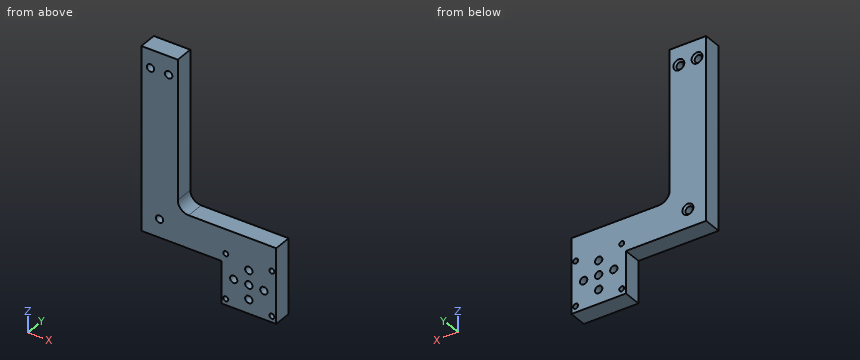
from build123d import *

# Parameters (mm, degrees)
BOSS_EXTRUDE1_DEPTH               = 12.7
F_1_4_20_TAPPED_HOLE1_D           = 5.1054
F_1_4_20_TAPPED_HOLE1_DEPTH       = 12.7
F_1_4_20_TAPPED_HOLE1_CSINK_D     = 7.62
F_1_4_20_TAPPED_HOLE1_CSINK_ANGLE = 90
F_1_4_20_TAPPED_HOLE2_D           = 5.1054
F_1_4_20_TAPPED_HOLE2_DEPTH       = 12.7
F_1_4_20_TAPPED_HOLE2_CSINK_D     = 7.62
F_1_4_20_TAPPED_HOLE2_CSINK_ANGLE = 90
F_29_0_136_DIAMETER_HOLE1_D       = 3.4544
F_29_0_136_DIAMETER_HOLE1_DEPTH   = 12.7
F_1_4_20_TAPPED_HOLE4_D           = 5.1054
F_1_4_20_TAPPED_HOLE4_DEPTH       = 12.7
LPATTERN1_COUNT                   = 3
LPATTERN1_PITCH                   = 10
F_1_4_20_TAPPED_HOLE6_D           = 5.1054
F_1_4_20_TAPPED_HOLE6_DEPTH       = 12.7
FILLET1_R                         = 7.62


with BuildPart() as part:
    # Sketch1 → Boss-Extrude1 (new body)
    with BuildSketch(Plane(origin=(0, 0, 0), x_dir=(1, 0, 0), z_dir=(0, 1, 0))):
        Polygon((81.28, 40.64), (81.28, 92.71), (43.18, 92.71), (43.18, 63.5), (12.7, 63.5), (-12.7, 63.5), (-12.7, -63.5), (12.7, -63.5), (12.7, 40.64), align=None)
    extrude(amount=BOSS_EXTRUDE1_DEPTH)

    # 1/4-20 Tapped Hole1
    with Locations(Plane(origin=(0, 12.7, 0), x_dir=(1, 0, 0), z_dir=(0, 1, 0))):
        with Locations((-6.35, -50.8), (6.35, -50.8)):
            CounterSinkHole(F_1_4_20_TAPPED_HOLE1_D / 2, F_1_4_20_TAPPED_HOLE1_CSINK_D / 2, depth=F_1_4_20_TAPPED_HOLE1_DEPTH, counter_sink_angle=F_1_4_20_TAPPED_HOLE1_CSINK_ANGLE)

    # 1/4-20 Tapped Hole2
    with Locations(Plane(origin=(0, 12.7, 0), x_dir=(1, 0, 0), z_dir=(0, 1, 0))):
        with Locations((0, 50.8)):
            CounterSinkHole(F_1_4_20_TAPPED_HOLE2_D / 2, F_1_4_20_TAPPED_HOLE2_CSINK_D / 2, depth=F_1_4_20_TAPPED_HOLE2_DEPTH, counter_sink_angle=F_1_4_20_TAPPED_HOLE2_CSINK_ANGLE)

    # #29 (0.136) Diameter Hole1
    with Locations(Plane(origin=(0, 12.7, 0), x_dir=(1, 0, 0), z_dir=(0, 1, 0))):
        with Locations((46.18, 88.44), (78.28, 88.44), (46.18, 57.44), (78.28, 57.44)):
            Hole(F_29_0_136_DIAMETER_HOLE1_D / 2, depth=F_29_0_136_DIAMETER_HOLE1_DEPTH)

    # 1/4-20 Tapped Hole4
    with Locations(Plane(origin=(0, 12.7, 0), x_dir=(1, 0, 0), z_dir=(0, 1, 0))):
        with Locations((62.23, 82.94)):
            f_1_4_20_tapped_hole4 = Hole(F_1_4_20_TAPPED_HOLE4_D / 2, depth=F_1_4_20_TAPPED_HOLE4_DEPTH)

    # LPattern1: 1/4-20 Tapped Hole4 ×3
    with Locations(*[(0, 0, i * LPATTERN1_PITCH) for i in range(1, LPATTERN1_COUNT)]):
        add(f_1_4_20_tapped_hole4, mode=Mode.SUBTRACT)

    # 1/4-20 Tapped Hole6
    with Locations(Plane(origin=(0, 12.7, 0), x_dir=(1, 0, 0), z_dir=(0, 1, 0))):
        with Locations((51.68, 72.972413119), (72.71230772, 72.972413119)):
            Hole(F_1_4_20_TAPPED_HOLE6_D / 2, depth=F_1_4_20_TAPPED_HOLE6_DEPTH)

    # Fillet1
    fillet1_edges = [part.edges().sort_by_distance(p)[0] for p in [
        (12.7, 6.35, -40.64),
    ]]
    fillet(fillet1_edges, radius=FILLET1_R)


solid = part.part
Geometry: final body of the model. Coordinates: model frame, mm. Coordinates: 2 decimals unless noted, no trailing zeros. Order: outer loops, then holes, each group sorted by start corner. A loop starts at its lowest first (then second) coordinate and runs counter-clockwise, first axis right, second up.
(1) Material intervals for probe 1 along X at (y, z) = (5, -57.44); probe 2 along Z at (x, y) = (62.5, 8.25); probe 3 along Z at (x, y) = (78.28, 7), sorted ascending.
(2) First-contact query: pin 1 (4.5 mm diameter, centred on x = 72.71, z = -72.97, fed in from -Y); pin 2 (6.5 mm diameter, centred on x = 25, y = 4.5, fed in from -Z); pin 3 (4 mm diameter, centred on x = 53, y = 7.5, fed in from +Z); pin 4 (6.5 mm diameter, centred on x = 6.35, z = 50.8, fed in from +Y). Flat tips, straight axial feed; report the tip coordinate or a pass-through.
(3) Section query C-C (x = -6.35). Return the cut outline in (y, z), plus the area to 3 significant figures.
(4) Section query B-B (x = 62.23). Return the cut outline in (y, z).
(5) Section query A-A (z = -88.44). Return the cut outline in (x, y), plus the area to 3 significant figures.
(6) Section query D-D (z = -57.44). Return the cut outline in (x, y).
Solution:
1. probe 1: x = -12.7 to 44.45, 47.91 to 76.55, 80.01 to 81.28
1. probe 2: z = -92.71 to -85.48, -80.4 to -75.48, -70.4 to -65.48, -60.4 to -40.64
1. probe 3: z = -92.71 to -90.17, -86.71 to -59.17, -55.71 to -40.64
2. pin 1: passes through
2. pin 2: stops at z = -63.5
2. pin 3: stops at z = -40.64
2. pin 4: stops at y = 12.14
3. outline: (0, -63.5) - (12.7, -63.5) - (12.7, 46.99) - (11.44, 48.25) - (0, 48.25) - close; (0, 53.35) - (11.44, 53.35) - (12.7, 54.61) - (12.7, 63.5) - (0, 63.5) - close
3. area: 1,550 mm2
4. outline: (0, -92.71) - (12.7, -92.71) - (12.7, -85.49) - (0, -85.49) - close; (0, -80.39) - (12.7, -80.39) - (12.7, -75.49) - (0, -75.49) - close; (0, -70.39) - (12.7, -70.39) - (12.7, -65.49) - (0, -65.49) - close; (0, -60.39) - (12.7, -60.39) - (12.7, -40.64) - (0, -40.64) - close
5. outline: (43.18, 0) - (44.45, 0) - (44.45, 12.7) - (43.18, 12.7) - close; (47.91, 0) - (76.55, 0) - (76.55, 12.7) - (47.91, 12.7) - close; (80.01, 0) - (81.28, 0) - (81.28, 12.7) - (80.01, 12.7) - close
5. area: 396 mm2
6. outline: (-12.7, 0) - (44.45, 0) - (44.45, 12.7) - (-12.7, 12.7) - close; (47.91, 0) - (76.55, 0) - (76.55, 12.7) - (47.91, 12.7) - close; (80.01, 0) - (81.28, 0) - (81.28, 12.7) - (80.01, 12.7) - close
